from build123d import *

# Parameters (mm, degrees)
SKETCH_1_W           = 35
SKETCH_1_H           = 55
EXTRUDE_1_DEPTH      = 1
EXTRUDE_2_DEPTH      = 3
SKETCH_3_R           = 5
CUT_EXTRUDE_1_DEPTH  = 169.569903897
SKETCH_4_R           = 4
CUT_EXTRUDE_2_DEPTH  = 2
SKETCH_5_R           = 2
CUT_EXTRUDE_3_DEPTH  = 2
EXTRUDE_START        = 7
EXTRUDE_3_DEPTH      = 7
CUT_EXTRUDE_START    = -1.5
SKETCH_9_W           = 10
SKETCH_9_H           = 26
CUT_EXTRUDE_4_DEPTH  = 168.318874833
SKETCH_10_R          = 1.5
CUT_EXTRUDE_5_DEPTH  = 194.595583627
SKETCH_11_W          = 338.377402865
SKETCH_11_H          = 318.232792562
CUT_EXTRUDE_6_DEPTH  = 10
SKETCH_12_W          = 33.023791835
SKETCH_12_H          = 7.5
CUT_EXTRUDE_7_DEPTH  = 74.963673636
CUT_EXTRUDE_START_2  = 9
CUT_EXTRUDE_8_DEPTH  = 10
EXTRUDE_START_2      = -2
EXTRUDE_4_DEPTH      = 2
EXTRUDE_5_DEPTH      = 8
SKETCH_16_R          = 1.5
CUT_EXTRUDE_9_DEPTH  = 53.962840747
SKETCH_17_R          = 1.75
CUT_EXTRUDE_10_DEPTH = 10
SKETCH_18_R          = 3
CUT_EXTRUDE_11_DEPTH = 1
FILLET_1_R           = 2
FILLET_2_R           = 2
FILLET_3_R           = 2
FILLET_4_R           = 2


with BuildPart() as part:
    # 草图1 → 凸台-拉伸1 (new body)
    with BuildSketch(Plane(origin=(0, 0, 0), x_dir=(1, 0, 0), z_dir=(0, 1, 0))):
        Rectangle(SKETCH_1_W, SKETCH_1_H)
    extrude(amount=EXTRUDE_1_DEPTH)

    # 草图2 → 凸台-拉伸2 (add)
    with BuildSketch(Plane(origin=(0, 1, 0), x_dir=(1, 0, 0), z_dir=(0, 1, 0))):
        with BuildLine():
            Line((106.75, -2.25), (106.75, 2.25))
            Line((106.75, 2.25), (121.75, 2.25))
            ThreePointArc((121.75, 2.25), (122.922125199, 2.352547667), (124.058635967, 2.65707481))
            Line((124.058635967, 2.65707481), (154.058635967, 13.576181838))
            ThreePointArc((154.058635967, 13.576181838), (158.397452333, 21.091232227), (151.75, 26.669107028))
            Line((151.75, 26.669107028), (-31.447415548, 57.101298968))
            ThreePointArc((-31.447415548, 57.101298968), (-37.800418235, 56.264673928), (-42.609265279, 52.029632639))
            Line((-42.609265279, 52.029632639), (-60.161792173, 23.605896086))
            ThreePointArc((-60.161792173, 23.605896086), (-61.717833724, 20.073278016), (-62.25, 16.25))
            Line((-62.25, 16.25), (-62.25, -16.25))
            ThreePointArc((-62.25, -16.25), (-61.717833724, -20.073278016), (-60.161792173, -23.605896086))
            Line((-60.161792173, -23.605896086), (-42.609265279, -52.029632639))
            ThreePointArc((-42.609265279, -52.029632639), (-37.800418235, -56.264673928), (-31.447415548, -57.101298968))
            Line((-31.447415548, -57.101298968), (151.75, -26.669107028))
            ThreePointArc((151.75, -26.669107028), (158.397452333, -21.091232227), (154.058635967, -13.576181838))
            Line((154.058635967, -13.576181838), (124.058635967, -2.65707481))
            ThreePointArc((124.058635967, -2.65707481), (122.922125199, -2.352547667), (121.75, -2.25))
            Line((121.75, -2.25), (106.75, -2.25))
        make_face()
    extrude(amount=EXTRUDE_2_DEPTH)

    # 草图3 → 切除-拉伸1 (cut, through all)
    with BuildSketch(Plane(origin=(0, 4, 0), x_dir=(1, 0, 0), z_dir=(0, 1, 0))):
        with Locations(Location((-48.25, 16.25, 0), (0, 0, 270))):
            Circle(SKETCH_3_R)
        with Locations(Location((-48.25, -16.25, 0), (0, 0, 270))):
            Circle(SKETCH_3_R)
    extrude(amount=-CUT_EXTRUDE_1_DEPTH, mode=Mode.SUBTRACT)

    # 草图4 → 切除-拉伸2 (cut)
    with BuildSketch(Plane(origin=(0, 4, 0), x_dir=(1, 0, 0), z_dir=(0, 1, 0))):
        with Locations(Location((-33.25, 46.25, 0), (0, 0, 270))):
            Circle(SKETCH_4_R)
        with Locations(Location((-33.25, -46.25, 0), (0, 0, 270))):
            Circle(SKETCH_4_R)
    extrude(amount=-CUT_EXTRUDE_2_DEPTH, mode=Mode.SUBTRACT)

    # 草图5 → 切除-拉伸3 (cut)
    with BuildSketch(Plane(origin=(0, 4, 0), x_dir=(1, 0, 0), z_dir=(0, 1, 0))):
        with Locations(Location((121.75, 9, 0), (0, 0, 270))):
            Circle(SKETCH_5_R)
        with Locations(Location((121.75, -9, 0), (0, 0, 270))):
            Circle(SKETCH_5_R)
        with Locations(Location((151.75, 19.919107028, 0), (0, 0, 270))):
            Circle(SKETCH_5_R)
        with Locations(Location((151.75, -19.919107028, 0), (0, 0, 270))):
            Circle(SKETCH_5_R)
    extrude(amount=-CUT_EXTRUDE_3_DEPTH, mode=Mode.SUBTRACT)

    # 草图8 → 凸台-拉伸3 (add)
    with BuildSketch(Plane.XZ.offset(-1).offset(EXTRUDE_START)):
        with BuildLine():
            Line((-26.75, -26.25), (-39.75, -26.25))
            Line((-39.75, -26.25), (-39.75, -55.124119675))
            ThreePointArc((-39.75, -55.124119675), (-35.798281322, -56.950759894), (-31.447415548, -57.101298968))
            Line((-31.447415548, -57.101298968), (-26.75, -56.320978726))
            Line((-26.75, -56.320978726), (-26.75, -26.25))
        make_face()
    extrude_3 = extrude(amount=-EXTRUDE_3_DEPTH)

    # 镜向1: 凸台-拉伸3 across plane
    add(extrude_3.mirror(Plane.XY))

    # 草图9 → 切除-拉伸4 (cut, through all)
    with BuildSketch(Plane.XZ.offset(6).offset(CUT_EXTRUDE_START)):
        with Locations((-33.25, -40.75)):
            Rectangle(SKETCH_9_W, SKETCH_9_H)
    cut_extrude_4 = extrude(amount=-CUT_EXTRUDE_4_DEPTH, mode=Mode.SUBTRACT)

    # 镜向2: 切除-拉伸4 across plane
    add(cut_extrude_4.mirror(Plane.XY), mode=Mode.SUBTRACT)

    # 草图10 → 切除-拉伸5 (cut, through all)
    with BuildSketch(Plane.XY.offset(-53.75)):
        with Locations((-33.25, -1.5)):
            Circle(SKETCH_10_R)
    cut_extrude_5 = extrude(amount=-CUT_EXTRUDE_5_DEPTH, mode=Mode.SUBTRACT)

    # 镜向3: 切除-拉伸5 across plane
    add(cut_extrude_5.mirror(Plane.XY), mode=Mode.SUBTRACT)

    # 草图11 → 切除-拉伸6 (cut)
    with BuildSketch(Plane.XZ.offset(6)):
        with Locations((33.683140033, 0)):
            Rectangle(SKETCH_11_W, SKETCH_11_H)
        with BuildLine():
            ThreePointArc((-30.464187664, 63.020189314), (-38.770685795, 62.328620225), (-45.75, 57.771718622))
            Line((-45.75, 57.771718622), (-45.75, 20.25))
            Line((-45.75, 20.25), (-20.75, 20.25))
            Line((-20.75, 20.25), (-20.75, 61.406498299))
            Line((-20.75, 61.406498299), (-30.464187664, 63.020189314))
        make_face(mode=Mode.SUBTRACT)
    extrude(amount=-CUT_EXTRUDE_6_DEPTH, mode=Mode.SUBTRACT)

    # 草图12 → 切除-拉伸7 (cut, through all)
    with BuildSketch(Plane(origin=(0, 4, 0), x_dir=(1, 0, 0), z_dir=(0, 1, 0))):
        with Locations((-37.261895917, -24)):
            Rectangle(SKETCH_12_W, SKETCH_12_H)
    extrude(amount=-CUT_EXTRUDE_7_DEPTH, mode=Mode.SUBTRACT)

    # 草图13 → 切除-拉伸8 (cut)
    with BuildSketch(Plane.XZ.offset(-1).offset(CUT_EXTRUDE_START_2)):
        Polygon((-26.75, 56.320978726), (-26.75, 27.75), (-20.75, 27.75), (-20.75, 55.324277157), align=None)
        with BuildLine():
            Line((-45.75, 46.943674541), (-45.75, 27.75))
            Line((-45.75, 27.75), (-39.75, 27.75))
            Line((-39.75, 27.75), (-39.75, 55.124119675))
            ThreePointArc((-39.75, 55.124119675), (-41.329172996, 53.715049478), (-42.609265279, 52.029632639))
            Line((-42.609265279, 52.029632639), (-45.75, 46.943674541))
        make_face()
    extrude(amount=-CUT_EXTRUDE_8_DEPTH, mode=Mode.SUBTRACT)

    # 草图14 → 凸台-拉伸4 (add)
    with BuildSketch(Plane(origin=(0, 4, 0), x_dir=(1, 0, 0), z_dir=(0, 1, 0)).offset(EXTRUDE_START_2)):
        with BuildLine():
            Line((-38.25, -53.75), (-38.25, -27.75))
            Line((-38.25, -27.75), (-45.75, -27.75))
            Line((-45.75, -27.75), (-45.75, -46.943674541))
            Line((-45.75, -46.943674541), (-42.609265279, -52.029632639))
            ThreePointArc((-42.609265279, -52.029632639), (-37.800418235, -56.264673928), (-31.447415548, -57.101298968))
            Line((-31.447415548, -57.101298968), (-20.75, -55.324277157))
            Line((-20.75, -55.324277157), (-20.75, -27.75))
            Line((-20.75, -27.75), (-28.25, -27.75))
            Line((-28.25, -27.75), (-28.25, -53.75))
            Line((-28.25, -53.75), (-38.25, -53.75))
        make_face()
        with BuildLine():
            Line((-20.75, -57.75), (-20.75, -55.324277157))
            Line((-20.75, -55.324277157), (-31.447415548, -57.101298968))
            ThreePointArc((-31.447415548, -57.101298968), (-37.800418235, -56.264673928), (-42.609265279, -52.029632639))
            Line((-42.609265279, -52.029632639), (-45.75, -46.943674541))
            Line((-45.75, -46.943674541), (-45.75, -57.75))
            Line((-45.75, -57.75), (-20.75, -57.75))
        make_face()
    extrude(amount=EXTRUDE_4_DEPTH)

    # 草图15 → 凸台-拉伸5 (add)
    with BuildSketch(Plane.XZ.offset(6)):
        with BuildLine():
            Line((-39.75, 55.124119675), (-39.75, 57.75))
            Line((-39.75, 57.75), (-26.75, 57.75))
            Line((-26.75, 57.75), (-26.75, 56.320978726))
            Line((-26.75, 56.320978726), (-31.447415548, 57.101298968))
            ThreePointArc((-31.447415548, 57.101298968), (-35.798281322, 56.950759894), (-39.75, 55.124119675))
        make_face()
    extrude(amount=-EXTRUDE_5_DEPTH)

    # 草图16 → 切除-拉伸9 (cut, through all)
    with BuildSketch(Plane(origin=(0, 0, 53.75), x_dir=(-1, 0, 0), z_dir=(0, 0, -1))):
        with Locations((33.25, -1.5)):
            Circle(SKETCH_16_R)
    extrude(amount=-CUT_EXTRUDE_9_DEPTH, mode=Mode.SUBTRACT)

    # 草图17 → 切除-拉伸10 (cut)
    with BuildSketch(Plane(origin=(0, 4, 0), x_dir=(1, 0, 0), z_dir=(0, 1, 0))):
        with Locations(Location((-24.25, -32.75, 0), (0, 0, 270))):
            Circle(SKETCH_17_R)
        with Locations(Location((-24.25, -42.75, 0), (0, 0, 270))):
            Circle(SKETCH_17_R)
        with Locations(Location((-42.25, -42.75, 0), (0, 0, 270))):
            Circle(SKETCH_17_R)
        with Locations(Location((-42.25, -32.75, 0), (0, 0, 270))):
            Circle(SKETCH_17_R)
    extrude(amount=-CUT_EXTRUDE_10_DEPTH, mode=Mode.SUBTRACT)

    # 草图18 → 切除-拉伸11 (cut)
    with BuildSketch(Plane(origin=(0, 4, 0), x_dir=(1, 0, 0), z_dir=(0, 1, 0))):
        with Locations(Location((-42.25, -32.75, 0), (0, 0, 270))):
            Circle(SKETCH_18_R)
        with Locations(Location((-24.25, -32.75, 0), (0, 0, 270))):
            Circle(SKETCH_18_R)
        with Locations(Location((-24.25, -42.75, 0), (0, 0, 270))):
            Circle(SKETCH_18_R)
        with Locations(Location((-42.25, -42.75, 0), (0, 0, 270))):
            Circle(SKETCH_18_R)
    extrude(amount=-CUT_EXTRUDE_11_DEPTH, mode=Mode.SUBTRACT)

    # 圆角1
    # the kernel refuses this fillet: 2 mm, written as the material it takes off along each edge
    with BuildSketch(Plane(origin=(-39.75, 2, 27.75), x_dir=(1, 0, 0), z_dir=(0, -1, 0))) as fillet_1_piece_1:
        with BuildLine():
            CenterArc((FILLET_1_R, FILLET_1_R), FILLET_1_R, 180, 90)
            Line((0, FILLET_1_R), (0, 0))
            Line((0, 0), (FILLET_1_R, 0))
        make_face()
    extrude(amount=13, mode=Mode.SUBTRACT)

    # 圆角2
    fillet_2_edges = [part.edges().sort_by_distance(p)[0] for p in [
        (-45.75, 3, 27.75),
        (-20.75, 3, 27.75),
    ]]
    fillet(fillet_2_edges, radius=FILLET_2_R)

    # 圆角3
    # the kernel refuses this fillet: 2 mm, written as the material it takes off along each edge
    with BuildSketch(Plane(origin=(-26.75, -11, 27.75), x_dir=(-1, 0, 0), z_dir=(0, 1, 0))) as fillet_3_piece_1:
        with BuildLine():
            CenterArc((FILLET_3_R, FILLET_3_R), FILLET_3_R, 180, 90)
            Line((0, FILLET_3_R), (0, 0))
            Line((0, 0), (FILLET_3_R, 0))
        make_face()
    extrude(amount=13, mode=Mode.SUBTRACT)

    # 圆角4
    fillet_4_edges = [part.edges().sort_by_distance(p)[0] for p in [
        (-28.25, -0.25, 53.75),
        (-38.25, -0.25, 53.75),
    ]]
    fillet(fillet_4_edges, radius=FILLET_4_R)


solid = part.part
Geometry: final body of the model. Coordinates: model frame, mm. A direction names the side the tool comes from. Coordinates: 2 decimals unless noted, no trailing zeros. Loops run counter-clockwise (first coordinate to the right, second up) from the corner with the lowest first, then second, coordinate; pieces in that order, holes last. Notation, with made-up numbers: (66, -25.5) - (116, -25.5) arc R23 cw to (116, -11.5) - close; hole circle Ø1 at (74, -14.75). An arc over 180 degrees is marked (long way). Put each result on its own line as item: value. Start each with the question number.
Q1. Cut plane B-B, the plane z = 42.75. Return loops of the section in (x, y).
Q2. Line query: line 1 (X direction, y = 3.55, z = 32.75); line 2 (X direction, y = 2.6, z = 42.75); line 3 (Y direction, x = -33.25, z = 56.55). Output: solid intervals per line, ascending.
Q3. Cut plane A-A, the plane x = -33.25. Return loops of the section in (y, z).
Q4. Set-up query: faces 1 (the cylindrical face through (-39.18, -1.94, 28.35)), 2 (the cylindrical face through (-37.65, -0.31, 53.18)), 3 (the cylindrical face through (-40.22, 3.51, 40.54)), 4 (the flat face through (-39.75, -2, 44)). Return all of +Z, -Z, +X, -X, +Y, -Y with unobstructed straight access to the full face (end or side cutting, diameter ignored); none if empty.
Q5. Cut plane C-C, the plane x = -42.25. Return loops of the section in (y, z), and give its area (3 significant figures).
Q6. Pin query (flat end, axial travel): pin 1 Ø3 at (x, y) = (-35.5, -0.5) entering from -Z; pin 2 Ø3 at (x, z) = (-24, 32) entering from +Y; pin 3 Ø2 at (x, z) = (-42.25, 32.75) entering from -Y; pin 4 Ø3 at (x, y) = (-34, -2) entering from -Z. Return the tip coordinate at first contact, or that it passes through.
Q7. Cut plane D-D, the plane y = -1.5. Return loops of the section in (x, z).
Filled sheet:
1. outline: (-45.75, 2) - (-44, 2) - (-44, 3) - (-45.25, 3) - (-45.25, 4) - (-45.75, 4) - close; (-40.5, 2) - (-39.75, 2) - (-39.75, -6) - (-26.75, -6) - (-26.75, 2) - (-26, 2) - (-26, 3) - (-27.25, 3) - (-27.25, 4) - (-28.25, 4) - (-28.25, -4.5) - (-38.25, -4.5) - (-38.25, 4) - (-39.25, 4) - (-39.25, 3) - (-40.5, 3) - close; (-22.5, 2) - (-20.75, 2) - (-20.75, 4) - (-21.25, 4) - (-21.25, 3) - (-22.5, 3) - close
2. line 1: -45.75 to -45.25, -39.25 to -38.25, -28.25 to -27.25, -21.25 to -20.75
2. line 2: -45.75 to -44, -40.5 to -38.25, -28.25 to -26, -22.5 to -20.75
2. line 3: -6 to -3, 0 to 4
3. outline: (-6, 27.75) - (-4.5, 27.75) - (-4.5, 53.75) - (-3, 53.75) - (-3, 57.75) - (-6, 57.75) - close; (0, 53.75) - (4, 53.75) - (4, 57.75) - (0, 57.75) - close
4. face 1: -Z, -X, -Y
4. face 2: -Z, +Y
4. face 3: +Y
4. face 4: +Z, -Z, -X, -Y
5. outline: (2, 27.75) - (4, 27.75) - (4, 29.75) - (3, 29.75) - (3, 31) - (2, 31) - close; (2, 34.5) - (3, 34.5) - (3, 35.75) - (4, 35.75) - (4, 39.75) - (3, 39.75) - (3, 41) - (2, 41) - close; (2, 44.5) - (3, 44.5) - (3, 45.75) - (4, 45.75) - (4, 57.75) - (2, 57.75) - close
5. area: 41.0 mm²
6. pin 1: z = 53.6
6. pin 2: y = 3
6. pin 3: through
6. pin 4: z = 53.75
7. outline: (-39.75, 29.75) arc R2 ccw to (-38.25, 27.81) - (-38.25, 51.75) arc R2 cw to (-36.25, 53.75) - (-34.75, 53.75) - (-34.75, 57.75) - (-39.75, 57.75) - close; (-31.75, 53.75) - (-30.25, 53.75) arc R2 cw to (-28.25, 51.75) - (-28.25, 27.81) arc R2 ccw to (-26.75, 29.75) - (-26.75, 57.75) - (-31.75, 57.75) - close
